Geometry check sheet. Reference: the model listing, model coordinates, mm. A direction names the side the tool comes from. Round coordinates to 2 decimals unless told otherwise and drop trailing zeros. Order: outer loops, then holes, each group sorted by start corner. A loop starts at its lowest first (then second) coordinate and runs counter-clockwise, first axis right, second up.
```python
from build123d import *

# Parameters (mm, degrees)
BASE_FLANGE_DEPTH          = 0.75
MOUNT_PEG_DEPTH            = 3
SKETCH4_W                  = 5
SKETCH4_H                  = 8.6
SCREW_BOSS_DEPTH           = 6
SCREW_BOSS_CHAMFER_DEPTH   = 8.6
SCREW_START                = -3
SCREW_BOSS_CLEARANCE_DEPTH = 36.87881814
M2_5_START                 = 1
M2_5_CLEARANCE_SLOT1_DEPTH = 3
PEG_CHAMFER_SIZE           = 0.5
FILLET1_R                  = 1
FILLET2_R                  = 4
SKETCH9_W                  = 5.5
SKETCH9_H                  = 16.180617206
CUT_EXTRUDE1_DEPTH         = 0.2
CHAMFER1_SIZE              = 0.692820323
CHAMFER1_SIZE_2            = 0.4


with BuildPart() as part:
    # Sketch1 → base flange (new body)
    with BuildSketch(Plane.XY):
        with BuildLine():
            Line((4, -24.677925359), (4, -9.442398166))
            ThreePointArc((4, -9.442398166), (-10.158758778, 1.399465338), (6.404113855, 8.009132841))
            Line((6.404113855, 8.009132841), (15.612630109, 19.525516154))
            ThreePointArc((15.612630109, 19.525516154), (-24.179534225, 6.352174798), (4, -24.677925359))
        make_face()
    extrude(amount=BASE_FLANGE_DEPTH)

    # Sketch3 → mount peg (add)
    with BuildSketch(Plane(origin=(0, 0, 0), x_dir=(-1, 0, 0), z_dir=(0, 0, -1))):
        with BuildLine():
            Line((9.575, -19), (9.575, -12))
            ThreePointArc((9.575, -12), (10.75, -10.825), (11.925, -12))
            Line((11.925, -12), (11.925, -19))
            ThreePointArc((11.925, -19), (10.75, -20.175), (9.575, -19))
        make_face()
    extrude(amount=MOUNT_PEG_DEPTH)

    # Sketch4 → screw boss (add)
    with BuildSketch(Plane.XY.offset(0.75)):
        with Locations((1.5, -17.060161762)):
            Rectangle(SKETCH4_W, SKETCH4_H)
    extrude(amount=SCREW_BOSS_DEPTH)

    # Sketch5 → screw boss chamfer (add)
    with BuildSketch(Plane.XZ.offset(21.360161762)):
        Polygon((-1, 0.75), (-1, 6.75), (-5, 0.75), align=None)
    extrude(amount=-SCREW_BOSS_CHAMFER_DEPTH)

    # Sketch6 → screw boss clearance (cut, through all)
    with BuildSketch(Plane(origin=(4, 0, 0), x_dir=(0, 0, -1), z_dir=(1, 0, 0)).offset(SCREW_START)):
        with BuildLine():
            Line((-6.75, -20.560161762), (-3.25, -20.560161762))
            ThreePointArc((-3.25, -20.560161762), (-1.835786438, -19.974375325), (-1.25, -18.560161762))
            Line((-1.25, -18.560161762), (-1.25, -15.560161762))
            ThreePointArc((-1.25, -15.560161762), (-1.835786438, -14.1459482), (-3.25, -13.560161762))
            Line((-3.25, -13.560161762), (-6.75, -13.560161762))
            Line((-6.75, -13.560161762), (-6.75, -20.560161762))
        make_face()
    extrude(amount=-SCREW_BOSS_CLEARANCE_DEPTH, mode=Mode.SUBTRACT)

    # M2.5 Clearance Slot1: read off the stored shape, not the designer's step
    # M2.5 Clearance Slot1 outline → M2.5 Clearance Slot1 (cut)
    with BuildSketch(Plane.YZ.offset(M2_5_START)):
        with BuildLine():
            ThreePointArc((-17.560161762, 5.45), (-19.010161762, 4), (-17.560161762, 2.55))
            Line((-17.560161762, 2.55), (-16.560161762, 2.55))
            ThreePointArc((-16.560161762, 2.55), (-15.110161762, 4), (-16.560161762, 5.45))
            Line((-16.560161762, 5.45), (-17.560161762, 5.45))
        make_face()
    extrude(amount=M2_5_CLEARANCE_SLOT1_DEPTH, mode=Mode.SUBTRACT)

    # M2.5 Clearance Slot1 2: loft between two sections, ruled curve by curve
    m2_5_clearance_slot1_2_from = [
        Edge.make_three_point_arc((2.327817459, -16.560161762, 5.45), (2.327817459, -15.53485693, 5.025304833), (2.327817459, -15.110161762, 4)),
        Edge.make_three_point_arc((2.327817459, -15.110161762, 4), (2.327817459, -15.53485693, 2.974695167), (2.327817459, -16.560161762, 2.55)),
        Edge.make_three_point_arc((2.327817459, -17.560161762, 2.55), (2.327817459, -18.585466595, 2.974695167), (2.327817459, -19.010161762, 4)),
        Edge.make_three_point_arc((2.327817459, -19.010161762, 4), (2.327817459, -18.585466595, 5.025304833), (2.327817459, -17.560161762, 5.45)),
        Edge.make_line((2.327817459, -16.560161762, 2.55), (2.327817459, -17.560161762, 2.55)),
        Edge.make_line((2.327817459, -16.560161762, 5.45), (2.327817459, -17.560161762, 5.45)),
    ]
    m2_5_clearance_slot1_2_to = [
        Edge.make_three_point_arc((1, -16.560161762, 6), (1, -15.1459482, 5.414213562), (1, -14.560161762, 4)),
        Edge.make_three_point_arc((1, -14.560161762, 4), (1, -15.1459482, 2.585786438), (1, -16.560161762, 2)),
        Edge.make_three_point_arc((1, -17.560161762, 2), (1, -18.974375325, 2.585786438), (1, -19.560161762, 4)),
        Edge.make_three_point_arc((1, -19.560161762, 4), (1, -18.974375325, 5.414213562), (1, -17.560161762, 6)),
        Edge.make_line((1, -16.560161762, 2), (1, -17.560161762, 2)),
        Edge.make_line((1, -16.560161762, 6), (1, -17.560161762, 6)),
    ]
    m2_5_clearance_slot1_2 = Solid(Shell([*[Face.make_surface_from_curves(m2_5_clearance_slot1_2_from[k], m2_5_clearance_slot1_2_to[k]) for k in range(6)], Face(Wire(m2_5_clearance_slot1_2_from)), Face(Wire(m2_5_clearance_slot1_2_to))]))
    add(m2_5_clearance_slot1_2, mode=Mode.SUBTRACT)

    # peg chamfer
    peg_chamfer_edges = [part.edges().sort_by_distance(p)[0] for p in [
        (-10.75, -20.175, -3),
        (-11.925, -15.5, -3),
        (-10.75, -10.825, -3),
        (-9.575, -15.5, -3),
    ]]
    chamfer(peg_chamfer_edges, length=PEG_CHAMFER_SIZE)

    # Fillet1
    fillet1_edges = [part.edges().sort_by_distance(p)[0] for p in [
        (-0.5, -12.760161762, 0.75),
        (-0.5, -21.360161762, 0.75),
        (-5, -17.060161762, 0.75),
    ]]
    fillet(fillet1_edges, radius=FILLET1_R)

    # Fillet2
    fillet2_edges = [part.edges().sort_by_distance(p)[0] for p in [
        (4, -9.442398166, 0.375),
        (4, -24.677925359, 0.375),
        (15.612630109, 19.525516154, 0.375),
        (6.404113855, 8.009132841, 0.375),
    ]]
    fillet(fillet2_edges, radius=FILLET2_R)

    # Sketch9 → Cut-Extrude1 (cut)
    with BuildSketch(Plane(origin=(0, 0, 0), x_dir=(-1, 0, 0), z_dir=(0, 0, -1))):
        with Locations((-1.25, -17.718085194)):
            Rectangle(SKETCH9_W, SKETCH9_H)
    extrude(amount=-CUT_EXTRUDE1_DEPTH, mode=Mode.SUBTRACT)

    # Chamfer1
    # the kernel refuses this chamfer: 0.692820323, 0.4 mm, written as the material it adds along each edge
    with BuildSketch(Plane(origin=(-1.5, -26.747345015, 0.2), x_dir=(1, 0, 0), z_dir=(0, 1, 0))) as chamfer1_piece_1_section:
        Polygon((CHAMFER1_SIZE, 0), (0, CHAMFER1_SIZE_2), (0, 0), align=None)
    chamfer1_piece_1 = extrude(amount=18.395329037, mode=Mode.PRIVATE)
    chamfer1_piece_1 = chamfer1_piece_1 & Plane(origin=(0, 0, 0.2), x_dir=(0.6245052043696531, 0.7810206461516994, 0), z_dir=(0, 0, -1)) * Cylinder(25, 40, mode=Mode.PRIVATE)
    chamfer1_piece_1 = chamfer1_piece_1 - Plane(origin=(0, 0, 0.2), x_dir=(0.39006502286727884, -0.9207873141695369, 0), z_dir=(0, 0, -1)) * Cylinder(10.254700538, 40, mode=Mode.PRIVATE)
    chamfer1_piece_1 = split(chamfer1_piece_1, bisect_by=Plane(origin=(-1.5, -26.747345015, 0), z_dir=(0, 0, 1)), keep=Keep.TOP, mode=Mode.PRIVATE)
    add(chamfer1_piece_1)


solid = part.part
```
(1) Set-up check for faces 1 (the cylindrical face through (-10.776, -20.175, -1.232)), 2 (the flat face through (-1, -20.56, 5)), 3 (the cylindrical face through (3.8, -13, 2.8)): record each of +Z, -Z, +X, -X, +Y, -Y from which the full face is reachable in a straight line by a thin tool's end or side.
Returned:
face 1: -Z, -Y
face 2: +Z, -X
face 3: +Z, -Z, +X
(2) Depth check by flat-ended pin: P1, Ø19.5, axis at x = 0.5, y = 1.5, coming from the -Z side; P2, Ø5.5, axis at x = 1, z = 5.5, coming from the -Y side; P3, Ø0.8, axis at y = -15, z = -1.5, coming from the +X side (3 decimals). Enter the tip coordinate at first touch or a pass-through.
Returned:
P1: stops at z = 0
P2: stops at y = -21.36
P3: stops at x = -9.575
(3) Material ranges on line 1 (Y direction, x = 0, z = 0.45); line 2 (Y direction, x = 0, z = 5.5); line 3 (X direction, y = 0, z = 0.65), recorded low to high.
Returned:
line 1: y = -25 to -10.25, 10.25 to 25
line 2: y = -21.36 to -20.56, -13.56 to -12.76
line 3: x = -25 to -10.25
(4) Sectioned sample at B-B, the plane y = 0. Record the cut outline in (x, z).
Returned:
outline: (-25, 0) - (-10.25, 0) - (-10.25, 0.75) - (-25, 0.75) - close
(5) Draft check along Y on faces 4 (the flat face through (3, -17, 2.55)), 5 (the cylindrical face through (-2, -14, 2)), 6 (the flat face through (4, -19, 3)), 7 (the flat face through (1, -12.76, 4)). Enter one of: released by +Y, released by -Y, zero draft, split by the parting line, or undercut.
Returned:
face 4: undercut
face 5: undercut
face 6: zero draft
face 7: released by +Y
(6) Sectioned sample at A-A, the plane x = -8. Record the cut outline in (y, z).
Returned:
outline: (-23.69, 0) - (-6.42, 0) - (-6.42, 0.75) - (-23.69, 0.75) - close; (6.42, 0) - (23.69, 0) - (23.69, 0.75) - (6.42, 0.75) - close
(7) Sectioned sample at C-C, the plane x = 7.5. Record the cut outline in (y, z).
Returned:
outline: (9.77, 0) - (23.85, 0) - (23.85, 0.75) - (9.77, 0.75) - close
